The figure shows three views and two pictorial views of one solid part (mm, origin at its lowest corner). Answer the questions. A direction names the side the tool comes from. Coordinates: 2 decimals unless noted, no trailing zeros. Order: outer loops, then holes, each group sorted by start corner. A loop starts at its lowest first (then second) coordinate and runs counter-clockwise, first axis right, second up. Notation, with made-up numbers: (36, 2.25) -> (68, 2.25) arc R28 cw to (68, 28.25) -> close; hole circle Ø5 at (-1.75, -25.75). An arc over 180 degrees is marked (long way). Write item = value, one per line. Start each with the question number.
Q1. The part is cut by section D-D, the plane y = 27. Determine the outline of the cut face in (x, z), plus the area to 3 significant figures.
Q2. The part is cut by section A-A, the plane z = 1.25. Determine the outline of the cut face in (x, y), plus the area to 3 significant figures.
Q3. For a pull along X with two mould halves and no side action, classify the marked faces 1, 2 and 3 as +X half, -X half, draft (parallel to the pull), parting line (faces both ways), or undercut.
Q4. Which of the six approach directions +Z, -Z, +X, -X, +Y, -Y give full straight-line access (tool end or side, diameter ignored) to the marked faces 4, 5 and 6?
Q5. The part is cut by section B-B, the plane x = 37.5. Determine the outline of the cut face in (y, z).
Q6. Straight lines are drawn through the part: L1, parallel to X at y = 25, z = 3; L2, parallel to Y at x = 37.5, z = 1.75; L3, parallel to Z at x = 12, y = 14. For each, find the intervals that lie inside material, in ascending order. Write a range as from..to.
Q7. The part is cut by section C-C, the plane z = 8.75. Determine the outline of the cut face in (x, y).
Q8. Flat-ended cylindrical pins translate along their axes: pin 1 (8.5 mm diameter, centred on x = 10.5, y = 39, fed in from -Z); pin 2 (2.5 mm diameter, centred on x = 18.5, z = 4.5, fed in from -Y); pin 3 (0.7 mm diameter, centred on y = 42, z = 9, fed in from +X); pin 4 (2 mm diameter, centred on y = 34.5, z = 4, fed in from -X). Find the tip coordinate at first contact, or state that the pin passes through.
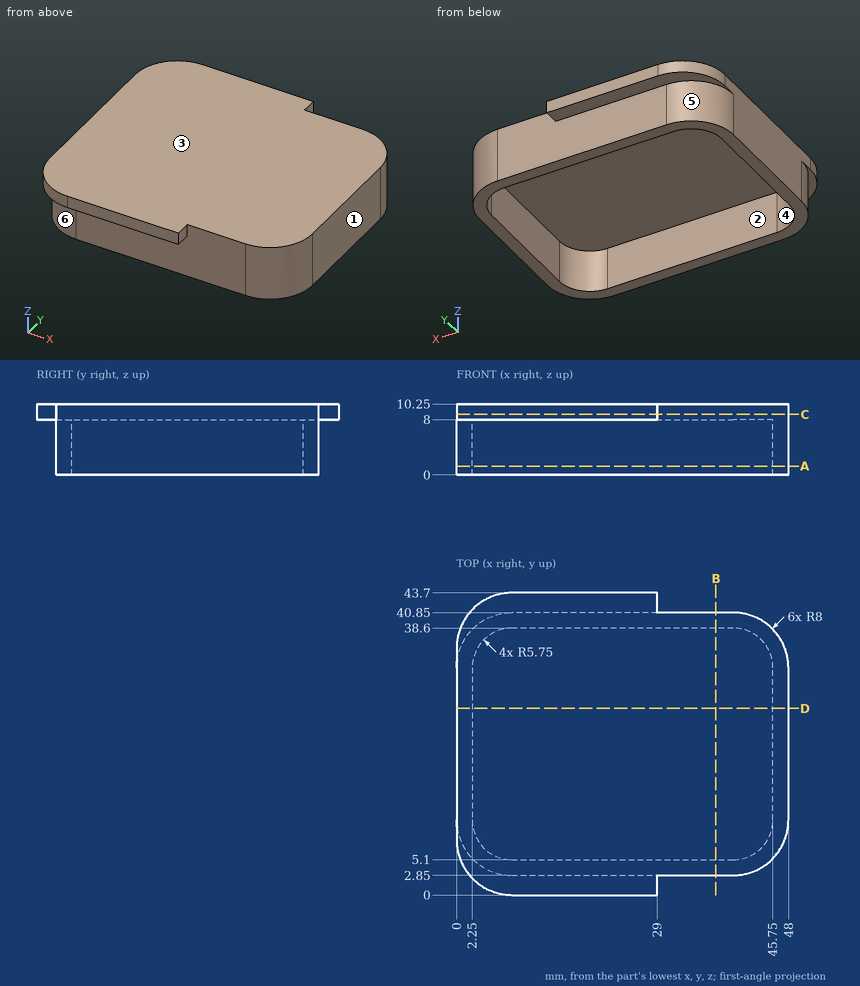
Model answer:
q1.outline = (0, 0) -> (2.25, 0) -> (2.25, 8) -> (45.75, 8) -> (45.75, 0) -> (48, 0) -> (48, 10.25) -> (0, 10.25) -> close
q1.area = 144 mm2
q2.outline = (0, 10.85) arc R8 ccw to (8, 2.85) -> (40, 2.85) arc R8 ccw to (48, 10.85) -> (48, 32.85) arc R8 ccw to (40, 40.85) -> (8, 40.85) arc R8 ccw to (0, 32.85) -> close; hole (2.25, 10.85) arc R5.75 ccw to (8, 5.1) -> (40, 5.1) arc R5.75 ccw to (45.75, 10.85) -> (45.75, 32.85) arc R5.75 ccw to (40, 38.6) -> (8, 38.6) arc R5.75 ccw to (2.25, 32.85) -> close
q2.area = 340 mm2
q3.face_1 = +X half
q3.face_2 = undercut
q3.face_3 = draft
q4.face_4 = -Z
q4.face_5 = -Z, -X, +Y
q4.face_6 = -Z, -X, -Y
q5.outline = (2.85, 0) -> (5.1, 0) -> (5.1, 8) -> (38.6, 8) -> (38.6, 0) -> (40.85, 0) -> (40.85, 10.25) -> (2.85, 10.25) -> close
q6.L1 = 0..2.25, 45.75..48
q6.L2 = 2.85..5.1, 38.6..40.85
q6.L3 = 8..10.25
q7.outline = (0, 8) arc R8 ccw to (8, 0) -> (29, 0) -> (29, 2.85) -> (40, 2.85) arc R8 ccw to (48, 10.85) -> (48, 32.85) arc R8 ccw to (40, 40.85) -> (29, 40.85) -> (29, 43.7) -> (8, 43.7) arc R8 ccw to (0, 35.7) -> close
q8.pin_1 = 0
q8.pin_2 = 2.85
q8.pin_3 = 29
q8.pin_4 = 0.03
